```python
from build123d import *

# Parameters (mm, degrees)
SKETCH1_R           = 1
BOSS_EXTRUDE1_DEPTH = 1


with BuildPart() as part:
    # Sketch1 → Boss-Extrude1 (new body)
    with BuildSketch(Plane.XY):
        with BuildLine():
            Line((-5, 17), (-1, 17))
            Line((-1, 17), (-1, 13.459935794))
            ThreePointArc((-1, 13.459935794), (0, -11.5), (1, 13.459935794))
            Line((1, 13.459935794), (1, 17))
            Line((1, 17), (5, 17))
            ThreePointArc((5, 17), (7.280116529, 13.941078138), (9.954900605, 11.22051487))
            ThreePointArc((9.954900605, 11.22051487), (0, -15), (-9.954900605, 11.22051487))
            ThreePointArc((-9.954900605, 11.22051487), (-7.280116529, 13.941078138), (-5, 17))
        make_face()
        with Locations((-2.5, 15.5)):
            Circle(SKETCH1_R, mode=Mode.SUBTRACT)
        with Locations(Location((2.5, 15.5, 0), (0, 0, 180))):
            Circle(SKETCH1_R, mode=Mode.SUBTRACT)
    extrude(amount=BOSS_EXTRUDE1_DEPTH)


solid = part.part
```
The listing builds one solid part. Answer for the finished solid, in the listing's coordinates (mm). A direction names the side the tool comes from. Give positions to 0.01 mm unless a question says otherwise; leave off trailing zeros. Loops run counter-clockwise (first coordinate to the right, second up) from the corner with the lowest first, then second, coordinate; pieces in that order, holes last. Notation, with made-up numbers: (57, 79.5) - (95, 79.5) arc R16 ccw to (95, 85.5) - close; hole circle Ø11 at (-0.5, 10). An arc over 180 degrees is marked (long way). Return JSON: item names as keys, results as strings. Group by question number.
1. Find section A-A (x = -9). Write down the section's boundary in (y, z), then the cut area to 3 significant figures.
2. Which of the six approach directions +Z, -Z, +X, -X, +Y, -Y give full straight-line access (tool end or side, diameter ignored) to faces 4 (the flat face through (-3, 17, 0.5)), 5 (the flat face through (1, 15.2, 0.5))?
3. Find section B-B (y = 0). Write down the section's boundary in (x, z), then the cut area to 3 significant figures.
4. Find section D-D (x = 2.5). Write down the section's boundary in (y, z), then the cut area to 3 significant figures.
5. Find section C-C (z = 0.45). Write down the section's boundary in (x, y), then the cut area to 3 significant figures.
6. Given pin 1 Ø5 at (x, y) = (9.5, -1.5) entering from -Z; pin 2 Ø0.5 at (y, z) = (14.5, 0.5) entering from -X; pin 3 Ø0.5 at (y, z) = (15, 0.5) entering from +X, each flat-ended and moving along its own axis, determine where each tip first touches the part or whether it passes through.
7. Straight lines are drawn through the part: line 1 (Y direction, x = -2.5, z = 0.4); line 2 (Y direction, x = 0, z = 0.6); line 3 (X direction, y = -2, z = 0.25). For each, find the intervals that lie inside material, in ascending order. Write a range as [from, to].
8. Determine the mould class of faces 1 (the flat face through (3, 17, 0.5)), 2 (the cylindrical face through (-2.717, 14.524, 0.493)), 3 (the flat face through (1, -12, 0)) for opening direction Y: pulls with the +Y half, pulls with the -Y half, needs draft (parallel to the pull), parting line crosses it, or undercut.
Verdict:
{
 "1": {"outline": "(-12, 0) - (-7.67, 0) - (-7.67, 1) - (-12, 1) - close; (9.67, 0) - (12.11, 0) - (12.11, 1) - (9.67, 1) - close", "area": "6.76 mm^2"},
 "2": {"face 4": "+Z, -Z, +X, -X, +Y", "face 5": "+Z, -Z, +Y"},
 "3": {"outline": "(-15, 0) - (-12.46, 0) - (-12.46, 1) - (-15, 1) - close; (12.46, 0) - (15, 0) - (15, 1) - (12.46, 1) - close", "area": "5.08 mm^2"},
 "4": {"outline": "(-14.79, 0) - (-11.25, 0) - (-11.25, 1) - (-14.79, 1) - close; (13.25, 0) - (14.5, 0) - (14.5, 1) - (13.25, 1) - close; (16.5, 0) - (17, 0) - (17, 1) - (16.5, 1) - close", "area": "5.30 mm^2"},
 "5": {"outline": "(-9.95, 11.22) arc R15 ccw (long way) to (9.95, 11.22) arc R28 cw to (5, 17) - (1, 17) - (1, 13.46) arc R12.5 cw (long way) to (-1, 13.46) - (-1, 17) - (-5, 17) arc R28 cw to start; hole circle Ø2 at (-2.5, 15.5); hole circle Ø2 at (2.5, 15.5)", "area": "235 mm^2"},
 "6": {"pin 1": "passes through", "pin 2": "stops at x = -7.02", "pin 3": "stops at x = 6.61"},
 "7": {"line 1": "y = [-14.79, -11.25], [13.25, 14.5], [16.5, 17]", "line 2": "y = [-15, -11.5]", "line 3": "x = [-14.87, -12.13], [12.13, 14.87]"},
 "8": {"face 1": "pulls with the +Y half", "face 2": "undercut", "face 3": "needs draft"}
}
